Part model, mm, in its own coordinate system. A direction names the side the tool comes from. Round coordinates to 2 decimals unless told otherwise and drop trailing zeros. Write each loop counter-clockwise with the first axis right and the second up, starting at its lowest first coordinate (ties: lowest second). Pieces come first, ordered by that corner, then holes. Notation, with made-up numbers: (79, 36.5) -> (83, 36.5) arc R22 cw to (83, 58.5) -> close; hole circle Ø2 at (46, -28). An arc over 180 degrees is marked (long way). Return JSON: item names as keys, results as strings. Group by question number.
```python
from build123d import *

# Parameters (mm, degrees)
SCHIZZO1_R                   = 28.525234369
ESTRUSIONE_ESTRUSIONE2_DEPTH = 5
SCHIZZO4_W                   = 10
SCHIZZO4_H                   = 6
TAGLIO_ESTRUSIONE1_DEPTH     = 5


with BuildPart() as part:
    # Schizzo1 → Estrusione-Estrusione2 (new, symmetric)
    with BuildSketch(Plane.XY):
        Circle(SCHIZZO1_R)
    extrude(amount=ESTRUSIONE_ESTRUSIONE2_DEPTH, both=True)

    # Schizzo4 → Taglio-Estrusione1 (cut, symmetric)
    with BuildSketch(Plane.XY.offset(5)):
        Rectangle(SCHIZZO4_W, SCHIZZO4_H)
    extrude(amount=TAGLIO_ESTRUSIONE1_DEPTH, both=True, mode=Mode.SUBTRACT)


solid = part.part
```
Item 1: Which spindle directions (+Z, -Z, +X, -X, +Y, -Y) get a long thin tool onto all of the face, cutting with end or side? Do faces 4 (the face through (0, 0, 0)), 5 (the face through (0, 0, -5)). Say none if no direction does.
Item 2: Cut at D-D (z = -3). Write the cut outline in (x, y), then the cut area to 3 significant figures.
Item 3: Cut at C-C (x = 0). Write the cut outline in (y, z).
Item 4: Cut at A-A (z = 3.75). Write the cut outline in (x, y), then the cut area to 3 significant figures.
Item 5: Flat gauge pins, fed straight in: P1, Ø4, axis at x = -1, z = 3.5, coming from the -Y side; P2, Ø1.5, axis at x = 8, z = 3.5, coming from the -Y side; P3, Ø5, axis at y = -6, z = -2, coming from the -X side. Where does each tip first touch, or does it go through?
Item 6: Cut at B-B (y = 0). Write the cut outline in (x, z), then the cut area to 3 significant figures.
Item 7: Wall check: L1, parallel to X at y = -1, z = 0.25; L2, parallel to Y at x = 13, z = -4; L3, parallel to Y at x = 19, z = 2.5. Give the ranges that are in metal, low to high.
Item 8: Two-plate mould, pull along X, no slides. Class faces 1 (the face through (0, -6, 5)), 2 (the face through (-28.498, 1.254, 0.07)), 3 (the face through (5, 0, 3)): released by +X, released by -X, zero draft, split by the parting line, or undercut.
Checks:
{
 "1": {"face 4": "+Z", "face 5": "-Z, +X, -X, +Y, -Y"},
 "2": {"outline": "circle Ø57.05 at (0, 0)", "area": "2,560 mm2"},
 "3": {"outline": "(-28.53, -5) -> (28.53, -5) -> (28.53, 5) -> (3, 5) -> (3, 0) -> (-3, 0) -> (-3, 5) -> (-28.53, 5) -> close"},
 "4": {"outline": "circle Ø57.05 at (0, 0); hole (-5, -3) -> (5, -3) -> (5, 3) -> (-5, 3) -> close", "area": "2,500 mm2"},
 "5": {"P1": "stops at y = -28.53", "P2": "stops at y = -27.59", "P3": "stops at x = -28.31"},
 "6": {"outline": "(-28.53, -5) -> (28.53, -5) -> (28.53, 5) -> (5, 5) -> (5, 0) -> (-5, 0) -> (-5, 5) -> (-28.53, 5) -> close", "area": "521 mm2"},
 "7": {"L1": "x = -28.51 to -5, 5 to 28.51", "L2": "y = -25.39 to 25.39", "L3": "y = -21.28 to 21.28"},
 "8": {"face 1": "zero draft", "face 2": "split by the parting line", "face 3": "undercut"}
}
